```python
from build123d import *

# Parameters (mm, degrees)
CHAMFER_1_SIZE         = 0.5
CHAMFER_2_SIZE         = 1
SKETCH_9_OUTSIDE_W     = 67.524
SKETCH_9_OUTSIDE_H     = 67.524
SKETCH_9_OUTSIDE_R     = 1.5
CUT_EXTRUDE_2_DEPTH    = 69.152402746
HOLE_WIZARD_M3_1_D     = 2.5
HOLE_WIZARD_M3_1_DEPTH = 5
HOLE_WIZARD_M3_1_TIP   = 0.751075774
HOLE_WIZARD_M3_2_D     = 2.5
HOLE_WIZARD_M3_2_DEPTH = 6.5
HOLE_WIZARD_M3_2_TIP   = 0.751075774
SKETCH_11_R            = 2.75
CUT_EXTRUDE_4_DEPTH    = 68.275504878


with BuildPart() as part:
    # 草图2 → 旋转1 (revolve)
    with BuildSketch(Plane.XY, mode=Mode.PRIVATE) as revolve_1_sk:
        Polygon((9, 2), (9, 7), (8.5, 7), (8.5, 37), (9, 37), (9, 42), (8.5, 42), (8.5, 59.5), (3.5, 59.5), (3.5, 51), (6.5, 48), (6.5, -5), (11.5, -5), (11.5, 0), (23.5, 0), (23.5, 2), align=None)
    revolve(revolve_1_sk.sketch.rotate(Axis((0, 0, 0), (0, 1, 0)), 90), axis=Axis((0, 0, 0), (0, 1, 0)))

    # 倒角1
    chamfer_1_edges = [part.edges().sort_by_distance(p)[0] for p in [
        (0, 7, 8.5),
        (0, 37, 8.5),
        (0, 42, 8.5),
    ]]
    chamfer(chamfer_1_edges, length=CHAMFER_1_SIZE - 0.0001)  # a hair under: the kernel refuses the full size

    # 倒角2
    chamfer_2_edges = [part.edges().sort_by_distance(p)[0] for p in [
        (0, 0, 11.5),
    ]]
    chamfer(chamfer_2_edges, length=CHAMFER_2_SIZE)

    # 草图9 outside → 切除-拉伸2 (cut, through all)
    # profile 1 of 4: a face of its own
    with BuildSketch(Plane.XZ):
        Rectangle(SKETCH_9_OUTSIDE_W, SKETCH_9_OUTSIDE_H)
        with BuildLine():
            Line((-3.031088913, 21.75), (-20.351596989, -8.25))
            ThreePointArc((-20.351596989, -8.25), (-20.351596989, -11.75), (-17.320508076, -13.5))
            Line((-17.320508076, -13.5), (17.320508076, -13.5))
            ThreePointArc((17.320508076, -13.5), (20.351596989, -11.75), (20.351596989, -8.25))
            Line((20.351596989, -8.25), (3.031088913, 21.75))
            ThreePointArc((3.031088913, 21.75), (0, 23.5), (-3.031088913, 21.75))
        make_face(mode=Mode.SUBTRACT)
    # profile 2 of 4: a face of its own
    with BuildSketch(Plane.XZ):
        with Locations(Location((0, 20, 0), (0, 0, 270))):
            Circle(SKETCH_9_OUTSIDE_R)
    # profile 3 of 4: a face of its own
    with BuildSketch(Plane.XZ):
        with Locations(Location((17.320508076, -10, 0), (0, 0, 270))):
            Circle(SKETCH_9_OUTSIDE_R)
    # profile 4 of 4: a face of its own
    with BuildSketch(Plane.XZ):
        with Locations(Location((-17.320508076, -10, 0), (0, 0, 270))):
            Circle(SKETCH_9_OUTSIDE_R)
    extrude(amount=-CUT_EXTRUDE_2_DEPTH, mode=Mode.SUBTRACT)

    # M3 螺纹孔1
    with Locations(Plane.XZ.offset(5)):
        with Locations((0, -9), (7.794228634, 4.5), (-7.794228634, 4.5)):
            Hole(HOLE_WIZARD_M3_1_D / 2, depth=HOLE_WIZARD_M3_1_DEPTH)
            with Locations((0, 0, -(HOLE_WIZARD_M3_1_DEPTH + HOLE_WIZARD_M3_1_TIP / 2))):  # 118° drill point
                Cone(0, HOLE_WIZARD_M3_1_D / 2, HOLE_WIZARD_M3_1_TIP, mode=Mode.SUBTRACT)

    # M3 螺纹孔2
    with Locations(Plane(origin=(0, 59.5, 0), x_dir=(1, 0, 0), z_dir=(0, 1, 0))):
        with Locations((0, 6), (5.196152423, -3), (-5.196152423, -3)):
            Hole(HOLE_WIZARD_M3_2_D / 2, depth=HOLE_WIZARD_M3_2_DEPTH)
            with Locations((0, 0, -(HOLE_WIZARD_M3_2_DEPTH + HOLE_WIZARD_M3_2_TIP / 2))):  # 118° drill point
                Cone(0, HOLE_WIZARD_M3_2_D / 2, HOLE_WIZARD_M3_2_TIP, mode=Mode.SUBTRACT)

    # 草图11 → 切除-拉伸4 (cut, through all)
    with BuildSketch(Plane.XY):
        with Locations(Location((0, 55, 0), (0, 0, 180))):
            Circle(SKETCH_11_R)
    extrude(amount=CUT_EXTRUDE_4_DEPTH, mode=Mode.SUBTRACT)


solid = part.part
```
Work out the finished part from the listing and answer in its coordinate system (mm). A direction names the side the tool comes from. Coordinates: 2 decimals unless noted, no trailing zeros. Write each loop counter-clockwise with the first axis right and the second up, starting at its lowest first coordinate (ties: lowest second). Pieces come first, ordered by that corner, then holes. Notation, with made-up numbers: (2, 83) - (57, 83) arc R23 ccw to (57, 101) - close; hole circle Ø1 at (11, 49.5). An arc over 180 degrees is marked (long way). Answer as a JSON object with one key per item and string values.
Q1. Consider L1, parallel to X at y = 1, z = -10; L2, parallel to X at y = -1, z = 4; L3, parallel to Y at x = -9, z = 5. Determine where each line is inside the solid, lowest interval first. Write a range as from..to.
Results list:
{"L1": "x = -20.82..-18.82, -15.82..15.82, 18.82..20.82", "L2": "x = -10.78..-8.94, -6.65..-5.12, 5.12..6.65, 8.94..10.78", "L3": "y = -5..2"}
Q2. Which of the six approach directions +Z, -Z, +X, -X, +Y, -Y give full straight-line access (tool end or side, diameter ignored) to faces 1 (the cylindrical face through (3.955, 21.129, 5.158)), 2 (the cylindrical face through (-8.428, 22.203, 1.107)), 3 (the cylindrical face through (0.27, 56.2, -4.78)), 4 (the flat face through (5, -5, 5)), 5 (the cylindrical face through (-1.05, 55.19, -3.34))?
Results list:
{"face 1": "-Y", "face 2": "none", "face 3": "+Y", "face 4": "+Z, -Z, +X, -X, -Y", "face 5": "+Y, -Y"}
Q3. Find section D-D (y = 6). Write down the section's boundary in (x, z), plus the area to 3 significant figures.
Results list:
{"outline": "circle Ø18 at (0, 0); hole circle Ø13 at (0, 0)", "area": "122 mm^2"}
Q4. Find section C-C (y = 29). Write down the section's boundary in (x, z), plus the area to 3 significant figures.
Results list:
{"outline": "circle Ø17 at (0, 0); hole circle Ø13 at (0, 0)", "area": "94.2 mm^2"}
Q5. Find section B-B (y = 55). Write down the section's boundary in (x, z), plus the area to 3 significant figures.
Results list:
{"outline": "(-2.75, 2.17) - (-2.75, 8.04) arc R8.5 ccw (long way) to (2.75, 8.04) - (2.75, 2.17) arc R3.5 cw (long way) to start; hole circle Ø2.5 at (-5.2, 3); hole circle Ø2.5 at (0, -6); hole circle Ø2.5 at (5.2, 3)", "area": "145 mm^2"}
Q6. For a pull along X with two mould halves and no side action, classify faces 6 (the cylindrical face through (-20.377, 0.986, -11.705)), 7 (the conical face through (0.12, 52.38, -6.18)), 8 (the cylindrical face through (-2.55, 51.12, -8.11)) as pulls with the +X half, pulls with the -X half, needs draft (parallel to the pull), parting line crosses it, or undercut.
Results list:
{"face 6": "pulls with the -X half", "face 7": "undercut", "face 8": "parting line crosses it"}
Q7. Given pin 1 Ø6 at (x, y) = (3.5, 19.5) entering from +Z; pin 2 Ø6 at (x, y) = (-6, 11.5) entering from +Z; pin 3 Ø1.5 at (x, z) = (-7.79, 4.5) entering from -Y, each flat-ended and moving along its own axis, determine where each tip first touches the part or whether it passes through.
Results list:
{"pin 1": "stops at z = 8.49", "pin 2": "stops at z = 7.95", "pin 3": "stops at y = 0.3"}
Q8. Find section A-A (z = 20). Write down the section's boundary in (x, y).
Results list:
{"outline": "(-4.04, 0) - (-1.5, 0) - (-1.5, 2) - (-4.04, 2) - close; (1.5, 0) - (4.04, 0) - (4.04, 2) - (1.5, 2) - close"}
